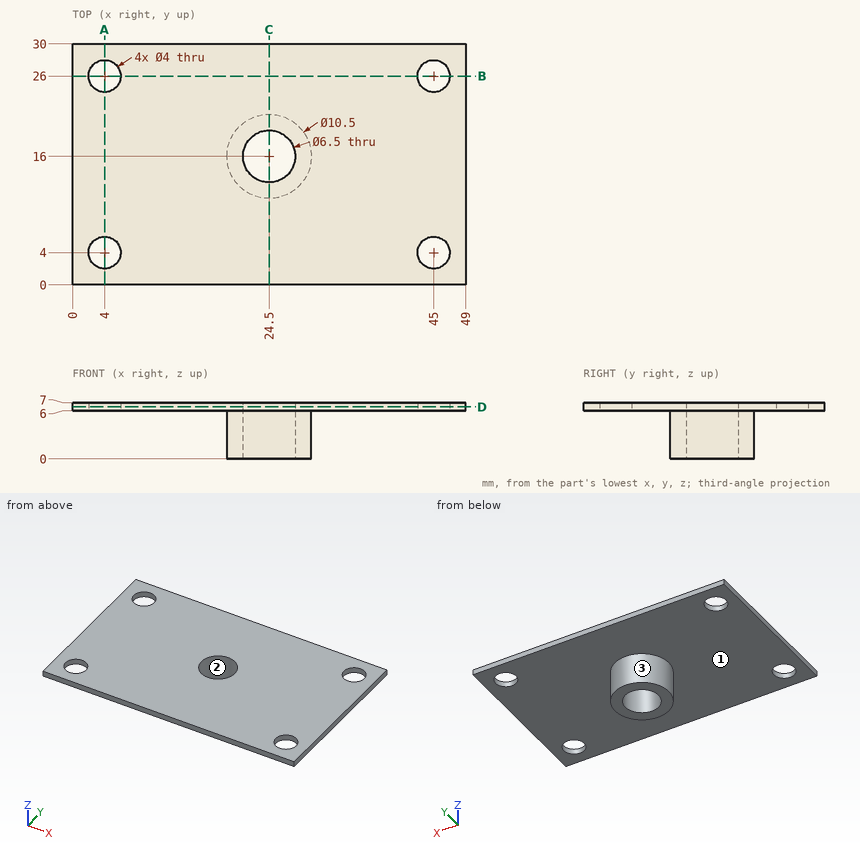
The drawing under review shows one solid part. Ordinate dimensions are in mm from its lowest x, y, z. Coordinates: 2 decimals unless noted, no trailing zeros. Order: outer loops, then holes, each group sorted by start corner. A loop starts at its lowest first (then second) coordinate and runs counter-clockwise, first axis right, second up. Notation, with made-up numbers: (74.5, 64.5) -> (97.5, 64.5) arc R14 ccw to (97.5, 78.5) -> close; hole circle Ø1 at (-20, -18.5). An arc over 180 degrees is marked (long way). Answer in a Markdown table with one row per item.
(1) Consider section C-C (x = 24.5). Write out the cut boundary in (y, z).
Answers:
| item | result |
|---|---|
| outline | (0, 6) -> (10.75, 6) -> (10.75, 0) -> (12.75, 0) -> (12.75, 7) -> (0, 7) -> close; (19.25, 0) -> (21.25, 0) -> (21.25, 6) -> (30, 6) -> (30, 7) -> (19.25, 7) -> close |
(2) Consider section A-A (x = 4). Write out the cut boundary in (y, z).
Answers:
| item | result |
|---|---|
| outline | (0, 6) -> (2, 6) -> (2, 7) -> (0, 7) -> close; (6, 6) -> (24, 6) -> (24, 7) -> (6, 7) -> close; (28, 6) -> (30, 6) -> (30, 7) -> (28, 7) -> close |
(3) Wall thickness on line 1 along Y through (x, z) = (45, 6.75); line 2 along X through (y, z) = (4, 6.45); line 3 along Z through (x, y) = (46.5, 13.75): over which ranges is each line inside the solid? List them lowest first.
Answers:
| item | result |
|---|---|
| line 1 | 0 to 2, 6 to 24, 28 to 30 |
| line 2 | 0 to 2, 6 to 43, 47 to 49 |
| line 3 | 6 to 7 |
(4) Insertion check: pin 1 (2.5 mm diameter, centred on x = 45, y = 26, fed in from -Z); pin 2 (1 mm diameter, centred on y = 21, z = 4.5, fed in from -X); pin 3 (6.5 mm diameter, centred on x = 4, y = 4, fed in from -Z); pin 4 (3 mm diameter, centred on x = 23, z = 1, fed in from +Y). Each pin has a flat end and moves straight along its axis. Give the tip position at first contact, or say it passes through.
Answers:
| item | result |
|---|---|
| pin 1 | through |
| pin 2 | x = 21.8 |
| pin 3 | z = 6 |
| pin 4 | y = 21.25 |
(5) Consider section D-D (z = 6.5). Write out the cut boundary in (x, y).
Answers:
| item | result |
|---|---|
| outline | (0, 0) -> (49, 0) -> (49, 30) -> (0, 30) -> close; hole circle Ø4 at (4, 4); hole circle Ø4 at (4, 26); hole circle Ø6.5 at (24.5, 16); hole circle Ø4 at (45, 4); hole circle Ø4 at (45, 26) |
(6) The part is to be moulded in two halves that separate along Y. For the marked faces 1, 2 and 3, say which applies: +Y half, -Y half, draft (parallel to the pull), parting line (faces both ways), or undercut.
Answers:
| item | result |
|---|---|
| face 1 | draft |
| face 2 | undercut |
| face 3 | parting line |
(7) Consider section B-B (y = 26). Write out the cut boundary in (x, z), plus the area to 3 significant figures.
Answers:
| item | result |
|---|---|
| outline | (0, 6) -> (2, 6) -> (2, 7) -> (0, 7) -> close; (6, 6) -> (43, 6) -> (43, 7) -> (6, 7) -> close; (47, 6) -> (49, 6) -> (49, 7) -> (47, 7) -> close |
| area | 41.0 mm² |
